The model under review builds one solid part; all positions refer to its coordinate system, in mm. A direction names the side the tool comes from. Round coordinates to 2 decimals unless told otherwise and drop trailing zeros. Order: outer loops, then holes, each group sorted by start corner. A loop starts at its lowest first (then second) coordinate and runs counter-clockwise, first axis right, second up.
```python
from build123d import *

# Parameters (mm, degrees)
F1_DEPTH = 3.81
F2_T     = -1.27
F3_R     = 1.524
F4_DEPTH = 25.4
F5_R     = 2.032
F6_DEPTH = 0.508
F7_R     = 1.27


with BuildPart() as f1:
    # F0 (on Top) → F1 (new body)
    with BuildSketch(Plane.XY):
        with BuildLine():
            ThreePointArc((22.86, 6.35), (22.116051, 8.146051), (20.32, 8.89))
            Line((20.32, 8.89), (-20.32, 8.89))
            ThreePointArc((-20.32, 8.89), (-22.116051, 8.146051), (-22.86, 6.35))
            Line((-22.86, 6.35), (-22.86, -6.35))
            ThreePointArc((-22.86, -6.35), (-22.116051, -8.146051), (-20.32, -8.89))
            Line((-20.32, -8.89), (20.32, -8.89))
            ThreePointArc((20.32, -8.89), (22.116051, -8.146051), (22.86, -6.35))
            Line((22.86, -6.35), (22.86, 6.35))
        make_face()
    extrude(amount=F1_DEPTH)

    # F2
    f2_openings = [f1.faces().sort_by_distance(p)[0] for p in [
        (0, 0, 3.81),
    ]]
    offset(amount=F2_T, openings=f2_openings)

    # F3 (on face) → F4 (cut)
    with BuildSketch(Plane.XY.offset(1.27)):
        with Locations((-12.7, 0)):
            Circle(F3_R)
        with Locations((-12.7, 50.8)):
            Circle(F3_R)
        Circle(F3_R)
        with Locations((0, 50.8)):
            Circle(F3_R)
        with Locations((12.7, 0)):
            Circle(F3_R)
        with Locations((12.7, 50.8)):
            Circle(F3_R)
    extrude(amount=-F4_DEPTH, mode=Mode.SUBTRACT)

    # F5 (on face) → F6 (cut)
    with BuildSketch(Plane.XY.offset(1.27)):
        with Locations((-12.7, 0)):
            Circle(F5_R)
        Circle(F5_R)
        with Locations((12.7, 0)):
            Circle(F5_R)
    extrude(amount=-F6_DEPTH, mode=Mode.SUBTRACT)

    # F7
    f7_edges = [f1.edges().sort_by_distance(p)[0] for p in [
        (0, -8.89, 0),
    ]]
    fillet(f7_edges, radius=F7_R)


solid = f1.part
```
(1) Consider section A-A (x = -12.7). Write out the cut boundary in (y, z), and give its area (3 significant figures).
Data:
outline: (-8.89, 1.27) arc R1.27 ccw to (-7.62, 0) - (-1.52, 0) - (-1.52, 0.76) - (-2.03, 0.76) - (-2.03, 1.27) - (-7.62, 1.27) - (-7.62, 3.81) - (-8.89, 3.81) - close; (1.52, 0) - (7.62, 0) arc R1.27 ccw to (8.89, 1.27) - (8.89, 3.81) - (7.62, 3.81) - (7.62, 1.27) - (2.03, 1.27) - (2.03, 0.76) - (1.52, 0.76) - close
area: 24.0 mm2
(2) Consider section C-C (y = 0). State how many separate pieces and enclosed holes the cut face has, and give its area (3 significant figures).
Data:
separate pieces: 4
enclosed holes: 0
area: 50.7 mm2
(3) To check wall thickness, follow probe 1 along Y at (x, z) = (-6.5, 1.95); probe 2 along X at (y, z) = (5.25, 1.7); probe 3 along Z at (x, y) = (5.5, -2.25). State the ranges of each line that lie inside material, in increasing order.
Data:
probe 1: y = -8.89 to -7.62, 7.62 to 8.89
probe 2: x = -22.86 to -21.59, 21.59 to 22.86
probe 3: z = 0 to 1.27
(4) Consider section B-B (z = 2.95). Write out the cut boundary in (x, y), and give its area (3 significant figures).
Data:
outline: (-22.86, -6.35) arc R2.54 ccw to (-20.32, -8.89) - (20.32, -8.89) arc R2.54 ccw to (22.86, -6.35) - (22.86, 6.35) arc R2.54 ccw to (20.32, 8.89) - (-20.32, 8.89) arc R2.54 ccw to (-22.86, 6.35) - close; hole (-21.59, -6.35) arc R1.27 ccw to (-20.32, -7.62) - (20.32, -7.62) arc R1.27 ccw to (21.59, -6.35) - (21.59, 6.35) arc R1.27 ccw to (20.32, 7.62) - (-20.32, 7.62) arc R1.27 ccw to (-21.59, 6.35) - close
area: 151 mm2
(5) Draft analysis for pull direction X (two halves, no side actions). For faces 3 (the flat face through (0, 7.62, 3)), 4 (the flat face through (-2, -8, 3.81)), 5 (the flat face through (22.86, 0, 3)), state which applies: pulls with the +X half, pulls with the -X half, needs draft (parallel to the pull), parting line crosses it, or undercut.
Data:
face 3: undercut
face 4: needs draft
face 5: pulls with the +X half
(6) Insertion check: pin 1 (5.5 mm diameter, centred on x = 0, y = 0, fed in from +Z); pin 2 (2.5 mm diameter, centred on x = 12.7, y = 0, fed in from +Z); pin 3 (3.5 mm diameter, centred on x = 12.7, y = 0, fed in from +Z). Each pin has a flat end and moves straight along its axis. Give the tip position at first contact, or say it passes through.
Data:
pin 1: stops at z = 1.27
pin 2: passes through
pin 3: stops at z = 0.76
(7) For faces 1 (the flat face through (11, 0, 0.762)), 2 (the flat face through (0, -8.89, 3)), list the 3-axis set-ups (+Z, -Z, +X, -X, +Y, -Y) from which the entire face can be reached by the end or side of a thin tool; tool diameter is ignored.
Data:
face 1: +Z
face 2: +Z, -Z, +X, -X, -Y
(8) Consider section D-D (y = -3). Write out the cut boundary in (x, z).
Data:
outline: (-22.86, 1.27) arc R1.27 ccw to (-21.59, 0) - (21.59, 0) arc R1.27 ccw to (22.86, 1.27) - (22.86, 3.81) - (21.59, 3.81) - (21.59, 1.27) - (-21.59, 1.27) - (-21.59, 3.81) - (-22.86, 3.81) - close
